The model under review builds one solid part; all positions refer to its coordinate system, in mm. A direction names the side the tool comes from. Coordinates: 2 decimals unless noted, no trailing zeros. Write each loop counter-clockwise with the first axis right and the second up, starting at its lowest first coordinate (ties: lowest second). Pieces come first, ordered by that corner, then holes. Notation, with made-up numbers: (35.25, 33.5) - (51.25, 33.5) arc R32 cw to (51.25, 65.5) - close; hole circle Ø11 at (37.25, 33). An arc over 180 degrees is marked (long way). Put each result on its own line as item: value.
from build123d import *

# Parameters (mm, degrees)
SKETCH014_W     = 9
SKETCH014_H     = 10
SKETCH014_R     = 2
PAD009_DEPTH    = 15
SKETCH015_R     = 1.75
POCKET002_DEPTH = 9.001
SKETCH016_R     = 3.72
POCKET003_DEPTH = 8


with BuildPart() as part:
    # Sketch014 → Pad009 (new body)
    with BuildSketch(Plane.XZ):
        with Locations((4.5, 5)):
            Rectangle(SKETCH014_W, SKETCH014_H)
        with Locations((4.5, 5)):
            Circle(SKETCH014_R, mode=Mode.SUBTRACT)
    extrude(amount=PAD009_DEPTH)

    # Sketch015 → Pocket002 (cut, through all)
    with BuildSketch(Plane.YZ):
        with Locations((-7.5, 5)):
            Circle(SKETCH015_R)
    extrude(amount=POCKET002_DEPTH, mode=Mode.SUBTRACT)

    # Sketch016 → Pocket003 (cut)
    with BuildSketch(Plane.YZ):
        with Locations((-7.5, 5)):
            Circle(SKETCH016_R)
    extrude(amount=POCKET003_DEPTH, mode=Mode.SUBTRACT)


solid = part.part
1. Consider section C-C on z = 5. State the section outline as (x, y) points.
Determined:
outline: (0, -15) - (2.5, -15) - (2.5, -11.22) - (0, -11.22) - close; (0, -3.78) - (2.5, -3.78) - (2.5, 0) - (0, 0) - close; (6.5, -15) - (9, -15) - (9, -9.25) - (8, -9.25) - (8, -11.22) - (6.5, -11.22) - close; (6.5, -3.78) - (8, -3.78) - (8, -5.75) - (9, -5.75) - (9, 0) - (6.5, 0) - close
2. For pin 1 Ø3.5 at (x, z) = (4.5, 5) entering from +Y; pin 2 Ø4.5 at (y, z) = (-7.5, 5) entering from -X, all flat-tipped, find the tip position at first contact; note any pin that passes through.
Determined:
pin 1: passes through
pin 2: stops at x = 8
3. Consider section A-A on y = -7.5. State the section outline as (x, z) points, plus the area to 3 significant figures.
Determined:
outline: (0, 0) - (9, 0) - (9, 3.25) - (8, 3.25) - (8, 1.28) - (0, 1.28) - close; (0, 8.72) - (8, 8.72) - (8, 6.75) - (9, 6.75) - (9, 10) - (0, 10) - close
area: 27.0 mm^2
4. Consider section B-B on x = 4.5. State the section outline as (y, z) points.
Determined:
outline: (-15, 0) - (0, 0) - (0, 3) - (-4.36, 3) arc R3.72 cw to (-10.64, 3) - (-15, 3) - close; (-15, 7) - (-10.64, 7) arc R3.72 cw to (-4.36, 7) - (0, 7) - (0, 10) - (-15, 10) - close
5. To check wall thickness, follow probe 1 along Y at (x, z) = (6.75, 5); probe 2 along Z at (x, y) = (4.5, -1.6); probe 3 along X at (y, z) = (-11.8, 5). State the ranges of each line that lie inside material, in increasing order.
Determined:
probe 1: y = -15 to -11.22, -3.78 to 0
probe 2: z = 0 to 3, 7 to 10
probe 3: x = 0 to 2.5, 6.5 to 9
6. Consider section D-D on y = -11.5. State the section outline as (x, z) points.
Determined:
outline: (0, 0) - (9, 0) - (9, 10) - (0, 10) - close; hole circle Ø4 at (4.5, 5)
7. The part is to be moulded in two halves that separate along Y. For faces 3 (the flat face through (2, -15, 5)), 4 (the cylindrical face through (3.944, -10.452, 2.736)), 5 (the flat face through (0, -11, 3)), 6 (the flat face through (2, 0, 5)), say which applies: +Y half, -Y half, draft (parallel to the pull), parting line (faces both ways), or undercut.
Determined:
face 3: -Y half
face 4: undercut
face 5: draft
face 6: +Y half
8. Machinability: for faces 1 (the flat face through (8, -7, 3)), 2 (the cylindrical face through (6.347, -12.788, 4.234)), which of the approach directions +Z, -Z, +X, -X, +Y, -Y give a long, thin tool a straight path to every point of the face, cutting with its end or side? Answer none if there is none.
Determined:
face 1: -X
face 2: +Y, -Y
